For this review, take the finished solid that the model builds, in its own axes (mm). Face numbers are marked on the shaded views. Coordinates: 2 decimals unless noted, no trailing zeros. Write each loop counter-clockwise with the first axis right and the second up, starting at its lowest first coordinate (ties: lowest second). Pieces come first, ordered by that corner, then holes.
1) Mouldability with a two-part tool opening along X and no side actions: class the marked faces 1, 2 and 3 as pulls with the +X half, pulls with the -X half, needs draft (parallel to the pull), parting line crosses it, or undercut.
2) To check wall thickness, follow line 1 along Y through (x, z) = (80, 5); line 2 along Y through (x, z) = (80, 10); line 3 along Y through (x, z) = (140.5, 23.5). State the ranges of each line that lie inside material, in increasing order.
3) We need section B-B on z = 22. Write out the cut boundary in (x, y).
4) We need section A-A on x = -80. Write out the cut boundary in (y, z).
5) We need section D-D on x = 59. Write out the cut boundary in (y, z).
6) Insertion check: P1, Ø5, axis at x = -49, z = 6.5, coming from the +Y side; P2, Ø1, axis at x = -42.5, y = 24, coming from the +Z side; P3, Ø9.5, axis at x = 80, y = -60, coming from the +Z side; P4, Ø5.5, axis at x = -80, y = -60, coming from the +Z side. Each pin has a flat end and moves straight along its axis. Give the tip position at first contact, or say it passes through.
7) We need section C-C on y = 35. Write out the cut boundary in (x, z), then the cut area to 3 significant figures.
from build123d import *

# Parameters (mm, degrees)
SCHIZZO1_W                   = 325
SCHIZZO1_H                   = 110
ESTRUSIONE_ESTRUSIONE1_DEPTH = 30
SCHIZZO2_W                   = 15
SCHIZZO2_H                   = 30
SCHIZZO2_W_2                 = 295
SCHIZZO2_H_2                 = 80
TAGLIO_ESTRUSIONE1_DEPTH     = 22
ESTRUSIONE_ESTRUSIONE2_START = -15
SCHIZZO3_W                   = 10
SCHIZZO3_H                   = 10
SCHIZZO3_R                   = 3
ESTRUSIONE_ESTRUSIONE2_DEPTH = 15
RACCORDO1_DEPTH              = 15
RACCORDO2_R                  = 4


with BuildPart() as part:
    # Schizzo1 → Estrusione-Estrusione1 (new body)
    with BuildSketch(Plane.XY):
        Rectangle(SCHIZZO1_W, SCHIZZO1_H)
    extrude(amount=ESTRUSIONE_ESTRUSIONE1_DEPTH)

    # Schizzo2 → Taglio-Estrusione1 (cut)
    with BuildSketch(Plane.XY.offset(30)):
        with Locations((155, 0)):
            Rectangle(SCHIZZO2_W, SCHIZZO2_H)
        Rectangle(SCHIZZO2_W_2, SCHIZZO2_H_2)
    extrude(amount=-TAGLIO_ESTRUSIONE1_DEPTH, mode=Mode.SUBTRACT)

    # Schizzo3 → Estrusione-Estrusione2 (add)
    # profile 1 of 4: a face of its own
    with BuildSketch(Plane.XY.offset(30).offset(ESTRUSIONE_ESTRUSIONE2_START)):
        with Locations((-80, 60)):
            Rectangle(SCHIZZO3_W, SCHIZZO3_H)
        with Locations((-80, 60)):
            Circle(SCHIZZO3_R, mode=Mode.SUBTRACT)
    # profile 2 of 4: a face of its own
    with BuildSketch(Plane.XY.offset(30).offset(ESTRUSIONE_ESTRUSIONE2_START)):
        with Locations((80, 60)):
            Rectangle(SCHIZZO3_W, SCHIZZO3_H)
        with Locations((80, 60)):
            Circle(SCHIZZO3_R, mode=Mode.SUBTRACT)
    # profile 3 of 4: a face of its own
    with BuildSketch(Plane.XY.offset(30).offset(ESTRUSIONE_ESTRUSIONE2_START)):
        with Locations((80, -60)):
            Rectangle(SCHIZZO3_W, SCHIZZO3_H)
        with Locations((80, -60)):
            Circle(SCHIZZO3_R, mode=Mode.SUBTRACT)
    # profile 4 of 4: a face of its own
    with BuildSketch(Plane.XY.offset(30).offset(ESTRUSIONE_ESTRUSIONE2_START)):
        with Locations((-80, -60)):
            Rectangle(SCHIZZO3_W, SCHIZZO3_H)
        with Locations((-80, -60)):
            Circle(SCHIZZO3_R, mode=Mode.SUBTRACT)
    extrude(amount=-ESTRUSIONE_ESTRUSIONE2_DEPTH)

    # Raccordo1: read off the stored shape, not the designer's step
    # Raccordo1 outline → Raccordo1 (add)
    with BuildSketch(Plane.XY):
        with BuildLine():
            Line((85, 55), (95, 55))
            add(Edge.make_bspline(
                [(95, 55), (85, 55), (85, 65)],
                knots=[0, 0, 0, 1, 1, 1], degree=2, weights=[1, 0.052631579, 1]))
            Line((85, 65), (85, 55))
        make_face()
        with BuildLine():
            Line((-95, 55), (-85, 55))
            Line((-85, 55), (-85, 65))
            add(Edge.make_bspline(
                [(-85, 65), (-85, 55), (-95, 55)],
                knots=[0, 0, 0, 1, 1, 1], degree=2, weights=[1, 0.052631579, 1]))
        make_face()
        with BuildLine():
            Line((-75, 55), (-65, 55))
            add(Edge.make_bspline(
                [(-65, 55), (-75, 55), (-75, 65)],
                knots=[0, 0, 0, 1, 1, 1], degree=2, weights=[1, 0.052631579, 1]))
            Line((-75, 65), (-75, 55))
        make_face()
        with BuildLine():
            Line((65, 55), (75, 55))
            Line((75, 55), (75, 65))
            add(Edge.make_bspline(
                [(75, 65), (75, 55), (65, 55)],
                knots=[0, 0, 0, 1, 1, 1], degree=2, weights=[1, 0.052631579, 1]))
        make_face()
        with BuildLine():
            Line((75, -55), (65, -55))
            add(Edge.make_bspline(
                [(65, -55), (75, -55), (75, -65)],
                knots=[0, 0, 0, 1, 1, 1], degree=2, weights=[1, 0.052631579, 1]))
            Line((75, -65), (75, -55))
        make_face()
        with BuildLine():
            Line((95, -55), (85, -55))
            Line((85, -55), (85, -65))
            add(Edge.make_bspline(
                [(85, -65), (85, -55), (95, -55)],
                knots=[0, 0, 0, 1, 1, 1], degree=2, weights=[1, 0.052631579, 1]))
        make_face()
        with BuildLine():
            Line((-85, -65), (-85, -55))
            Line((-85, -55), (-95, -55))
            add(Edge.make_bspline(
                [(-95, -55), (-85, -55), (-85, -65)],
                knots=[0, 0, 0, 1, 1, 1], degree=2, weights=[1, 0.052631579, 1]))
        make_face()
        with BuildLine():
            add(Edge.make_bspline(
                [(-75, -65), (-75, -55), (-65, -55)],
                knots=[0, 0, 0, 1, 1, 1], degree=2, weights=[1, 0.052631579, 1]))
            Line((-65, -55), (-75, -55))
            Line((-75, -55), (-75, -65))
        make_face()
    extrude(amount=RACCORDO1_DEPTH)

    # Raccordo2
    raccordo2_edges = [part.edges().sort_by_distance(p)[0] for p in [
        (0, 40, 30),
        (-147.5, 0, 30),
        (0, -40, 30),
        (147.5, -27.5, 30),
        (155, -15, 30),
        (162.5, -35, 30),
        (0, -55, 30),
        (-162.5, 0, 30),
        (0, 55, 30),
        (162.5, 35, 30),
        (155, 15, 30),
        (147.5, 27.5, 30),
        (-162.5, 55, 15),
        (-162.5, -55, 15),
        (162.5, -55, 15),
        (162.5, 55, 15),
    ]]
    fillet(raccordo2_edges, radius=RACCORDO2_R)


solid = part.part
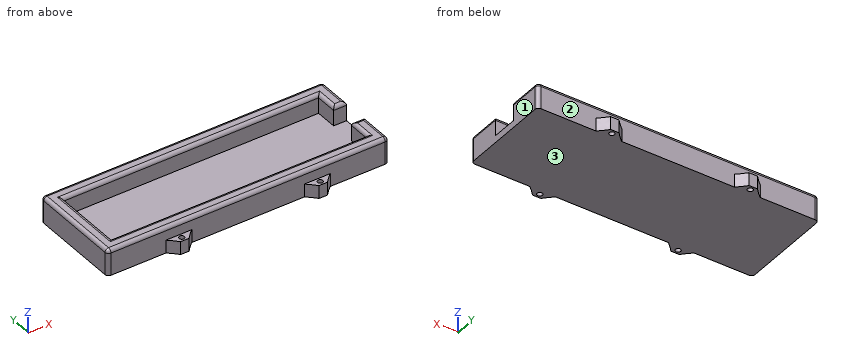
Result:
1. face 1: pulls with the +X half
1. face 2: undercut
1. face 3: needs draft
2. line 1: y = -65 to -63, -57 to 57, 63 to 65
2. line 2: y = -65 to -63, -57 to -40, 40 to 57, 63 to 65
2. line 3: y = -55 to -40, 40 to 55
3. outline: (-162.5, -51) arc R4 ccw to (-158.5, -55) - (158.5, -55) arc R4 ccw to (162.5, -51) - (162.5, -15) - (147.5, -15) - (147.5, -40) - (-147.5, -40) - (-147.5, 40) - (147.5, 40) - (147.5, 15) - (162.5, 15) - (162.5, 51) arc R4 ccw to (158.5, 55) - (-158.5, 55) arc R4 ccw to (-162.5, 51) - close
4. outline: (-65, 0) - (-63, 0) - (-63, 15) - (-65, 15) - close; (-57, 0) - (57, 0) - (57, 15) - (55, 15) - (55, 26) arc R4 ccw to (51, 30) - (44, 30) arc R4 ccw to (40, 26) - (40, 8) - (-40, 8) - (-40, 26) arc R4 ccw to (-44, 30) - (-51, 30) arc R4 ccw to (-55, 26) - (-55, 15) - (-57, 15) - close; (63, 0) - (65, 0) - (65, 15) - (63, 15) - close
5. outline: (-55, 0) - (55, 0) - (55, 26) arc R4 ccw to (51, 30) - (44, 30) arc R4 ccw to (40, 26) - (40, 8) - (-40, 8) - (-40, 26) arc R4 ccw to (-44, 30) - (-51, 30) arc R4 ccw to (-55, 26) - close
6. P1: stops at y = 55
6. P2: stops at z = 8
6. P3: stops at z = 15
6. P4: passes through
7. outline: (-162.5, 0) - (162.5, 0) - (162.5, 26) arc R4 ccw to (158.5, 30) - (151.5, 30) arc R4 ccw to (147.5, 26) - (147.5, 8) - (-147.5, 8) - (-147.5, 26) arc R4 ccw to (-151.5, 30) - (-158.5, 30) arc R4 ccw to (-162.5, 26) - close
7. area: 3,250 mm2
